```python
from build123d import *

# Parameters (mm, degrees)
F1_DEPTH = 63.5
F0_W     = 25.4
F0_H     = 5.715
F0_H_2   = 3.81
F0_H_3   = 19.05
F2_DEPTH = 25.4
F3_DEPTH = 9.525
F5_R     = 6.35


with BuildPart() as f1:
    # F0 (on Front) → F1 (new body, symmetric)
    with BuildSketch(Plane.XZ):
        Polygon((22.225, 9.525), (-41.275, 9.525), (-41.275, -9.525), (41.275, -9.525), (41.275, 9.525), align=None)
    extrude(amount=F1_DEPTH, both=True)

    # F0 (on Front) → F2 (join, symmetric)
    with BuildSketch(Plane.XZ):
        with BuildLine():
            Line((22.225, 27.94), (22.225, 9.525))
            Line((22.225, 9.525), (41.275, 9.525))
            Line((41.275, 9.525), (41.275, 27.94))
            ThreePointArc((41.275, 27.94), (45.9246798487, 39.1653201513), (57.15, 43.815))
            Line((57.15, 43.815), (60.325, 43.815))
            Line((60.325, 43.815), (60.325, 62.865))
            Line((60.325, 62.865), (57.15, 62.865))
            add(Edge.make_bspline(
                [(53.8414351699, 62.7079309676), (54.9353913903, 62.7725296007), (56.0381901925, 62.8249247758), (57.15, 62.865)],
                knots=[109.0590899765, 109.0590899765, 109.0590899765, 109.0590899765, 111.9492573669, 111.9492573669, 111.9492573669, 111.9492573669], degree=3))
            ThreePointArc((53.8414351699, 62.7079309676), (31.3110057114, 51.4368508348), (22.225, 27.94))
        make_face()
        with Locations((73.025, 40.9575)):
            Rectangle(F0_W, F0_H)
        with Locations((73.025, 64.77)):
            Rectangle(F0_W, F0_H_2)
        with Locations((73.025, 53.34)):
            Rectangle(F0_W, F0_H_3)
    extrude(amount=F2_DEPTH, both=True)

    # F0 (on Front) → F3 (join, symmetric)
    with BuildSketch(Plane.XZ):
        with BuildLine():
            add(Edge.make_bspline(
                [(-41.275, 9.525), (-16.1274971076, 40.4562996606), (12.5615182112, 60.2703323134), (53.8414351699, 62.7079309676)],
                knots=[0, 0, 0, 0, 109.0590899765, 109.0590899765, 109.0590899765, 109.0590899765], degree=3))
            Line((-41.275, 9.525), (22.225, 9.525))
            Line((22.225, 9.525), (22.225, 27.94))
            ThreePointArc((22.225, 27.94), (31.3110057114, 51.4368508348), (53.8414351699, 62.7079309676))
        make_face()
    extrude(amount=F3_DEPTH, both=True)

    # F0 (on Front) → F4 (revolve)
    with BuildSketch(Plane.XZ):
        Polygon((85.725, 66.675), (85.725, 62.865), (85.725, 43.815), (85.725, 38.1), (111.125, 38.1), (111.125, 66.675), align=None)
    revolve(axis=Axis((85.725, 0, 52.3875), (0, 0, 1)))

    # F5
    f5_edges = [f1.edges().sort_by_distance(p)[0] for p in [
        (-41.275, 63.5, 0),
        (41.275, 63.5, 0),
        (41.275, -63.5, 0),
        (-41.275, -63.5, 0),
    ]]
    fillet(f5_edges, radius=F5_R)


solid = f1.part
```
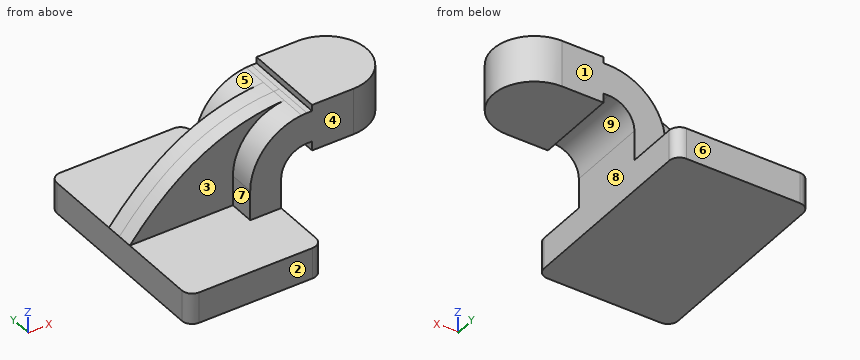
Here's how the part is built. I have some questions about the finished solid (model axes, mm). Face numbers are marked on the shaded views. A direction names the side the tool comes from. Round coordinates to 2 decimals unless told otherwise and drop trailing zeros. Loops run counter-clockwise (first coordinate to the right, second up) from the corner with the lowest first, then second, coordinate; pieces in that order, holes last.
1. Suppose I cut it at C-C, the plane x = 101. Please give me the cut outline in (y, z) (3 decimals), and give its area (3 significant figures).
Answers:
outline: (-20.294, 38.1) - (20.294, 38.1) - (20.294, 66.675) - (-20.294, 66.675) - close
area: 1,160 mm2
2. For the marked faces 1, 2, 3, 4 and 5, which set-ups out of +Z, -Z, +X, -X, +Y, -Y let a thin tool reach every point of the face, with its end or its side?
Answers:
face 1: +Z, +X, -X, +Y
face 2: +Z, -Z, +X, -X, -Y
face 3: +Z, -X, -Y
face 4: +Z, +X, -X, -Y
face 5: +Z, -X, +Y
3. If I drill on probe 1 along Z at (x, y) = (-20.5, 31.5) (3 decimals); probe 2 along X at (y, z) = (-17, 14) (3 decimals); probe 3 along Y at (x, z) = (26.5, 31.5), over which ranges is the centre line in solid material (lowest first)?
Answers:
probe 1: z = -9.525 to 9.525
probe 2: x = 22.225 to 41.275
probe 3: y = -25.4 to 25.4
4. Suppose I cut it at A-A, the plane z = -0.5. Please give me the cut outline in (x, y) (3 decimals).
Answers:
outline: (-41.275, -57.15) arc R6.35 ccw to (-34.925, -63.5) - (34.925, -63.5) arc R6.35 ccw to (41.275, -57.15) - (41.275, 57.15) arc R6.35 ccw to (34.925, 63.5) - (-34.925, 63.5) arc R6.35 ccw to (-41.275, 57.15) - close
5. Thinking about a two-plate mould opening in X: for the marked faces 6, 7, 8 and 9, which applies, released by +X, released by -X, zero draft, split by the parting line, or undercut?
Answers:
face 6: zero draft
face 7: released by -X
face 8: released by +X
face 9: undercut
6. Suppose I cut it at B-B, the plane y = -30.5. Please give me the cut outline in (x, z) (3 decimals).
Answers:
outline: (-41.275, -9.525) - (41.275, -9.525) - (41.275, 9.525) - (-41.275, 9.525) - close
7. Will these pins go through, and if not, where does the flat tip stop? pin 1 (8 mm diameter, centred on y = 15.5, z = 16, fed in from -X) (3 decimals); pin 2 (1.7 mm diameter, centred on y = -4, z = 42, fed in from -X); pin 3 (16 mm diameter, centred on x = 10.5, z = 41, fed in from +Y) (3 decimals).
Answers:
pin 1: stops at x = 22.225
pin 2: stops at x = -8.48
pin 3: stops at y = 9.525
